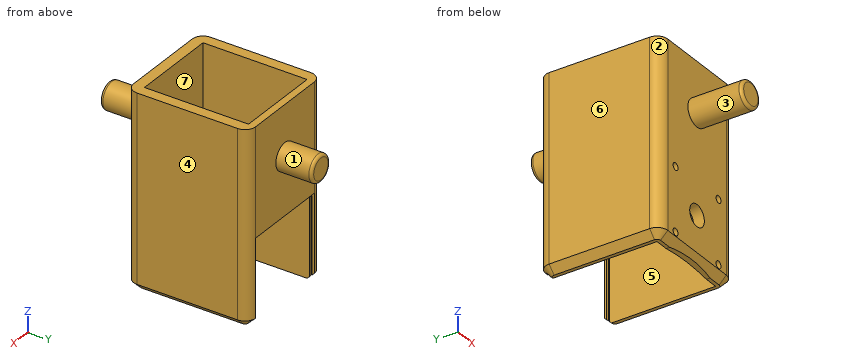
```python
from build123d import *

# Parameters (mm, degrees)
BOSS_EXTRUDE1_DEPTH = 69.85
CUT_EXTRUDE1_DEPTH  = 50.8
SKETCH3_R           = 1.27
SKETCH3_R_2         = 3.81
CUT_EXTRUDE2_DEPTH  = 50.8
SKETCH4_W           = 30.48
SKETCH4_H           = 38.1
BOSS_EXTRUDE2_DEPTH = 2.54
SKETCH5_W           = 30.48
SKETCH5_H           = 1.016
CUT_EXTRUDE3_DEPTH  = 1.016
FILLET1_R           = 3.81
SKETCH6_R           = 4.7625
BOSS_EXTRUDE3_DEPTH = 12.7
BOSS_EXTRUDE4_START = 19.05
SKETCH8_R           = 4.7625
BOSS_EXTRUDE4_DEPTH = 19.05
FILLET2_R           = 1.016
SKETCH9_W           = 38.1
SKETCH9_H           = 43.18
CUT_EXTRUDE4_DEPTH  = 2.032


# Some blends are built 0.0001 mm under size
with BuildPart() as part:
    # Sketch1 → Boss-Extrude1 (new body)
    with BuildSketch(Plane.XY):
        Polygon((15.24, -19.685), (-15.24, -19.685), (-15.24, 19.685), (-19.05, 19.685), (-19.05, -23.495), (15.24, -23.495), (19.05, -23.495), (19.05, 19.685), (15.24, 19.685), align=None)
    extrude(amount=BOSS_EXTRUDE1_DEPTH)

    # Sketch2 → Cut-Extrude1 (cut)
    with BuildSketch(Plane(origin=(0, 19.685, 0), x_dir=(1, 0, 0), z_dir=(0, 1, 0))):
        with BuildLine():
            Line((-19.05, 0), (19.05, 0))
            ThreePointArc((19.05, 0), (0, -2.54), (-19.05, 0))
        make_face()
    extrude(amount=-CUT_EXTRUDE1_DEPTH, mode=Mode.SUBTRACT)

    # Sketch3 → Cut-Extrude2 (cut)
    with BuildSketch(Plane(origin=(0, 19.685, 0), x_dir=(1, 0, 0), z_dir=(0, 1, 0))):
        with Locations(Location((-11.176, -5.842, 0), (0, 0, 270))):
            Circle(SKETCH3_R)
        with Locations(Location((11.176, -5.842, 0), (0, 0, 270))):
            Circle(SKETCH3_R)
        with Locations(Location((11.176, -28.194, 0), (0, 0, 270))):
            Circle(SKETCH3_R)
        with Locations(Location((-11.176, -28.194, 0), (0, 0, 270))):
            Circle(SKETCH3_R)
        with Locations(Location((0, -17.018, 0), (0, 0, 270))):
            Circle(SKETCH3_R_2)
    extrude(amount=-CUT_EXTRUDE2_DEPTH, mode=Mode.SUBTRACT)

    # Sketch4 → Boss-Extrude2 (add)
    with BuildSketch(Plane(origin=(0, 19.685, 0), x_dir=(1, 0, 0), z_dir=(0, 1, 0))):
        with Locations((0, -50.8)):
            Rectangle(SKETCH4_W, SKETCH4_H)
    extrude(amount=-BOSS_EXTRUDE2_DEPTH)

    # Sketch5 → Cut-Extrude3 (cut)
    with BuildSketch(Plane(origin=(-15.24, 0, 0), x_dir=(0, 0, -1), z_dir=(1, 0, 0))):
        with Locations((-15.24, 18.415)):
            Rectangle(SKETCH5_W, SKETCH5_H)
    cut_extrude3 = extrude(amount=-CUT_EXTRUDE3_DEPTH, mode=Mode.SUBTRACT)

    # Mirror1: Cut-Extrude3 across plane
    add(cut_extrude3.mirror(Plane(origin=(0, 0, 0), x_dir=(0, 0, 1), z_dir=(1, 0, 0))), mode=Mode.SUBTRACT)

    # Fillet1
    fillet1_edges = [part.edges().sort_by_distance(p)[0] for p in [
        (19.05, 19.685, 34.925),
        (19.05, -23.495, 34.925),
        (-19.05, -23.495, 34.925),
        (-19.05, 19.685, 34.925),
    ]]
    fillet(fillet1_edges, radius=FILLET1_R - 0.0001)  # a hair under: the kernel refuses the full size

    # Sketch6 → Boss-Extrude3 (add)
    with BuildSketch(Plane(origin=(0, 19.685, 0), x_dir=(1, 0, 0), z_dir=(0, 1, 0))):
        with Locations((0, -52.07)):
            Circle(SKETCH6_R)
    extrude(amount=BOSS_EXTRUDE3_DEPTH)

    # Sketch8 → Boss-Extrude4 (add)
    with BuildSketch(Plane.XZ.offset(23.495).offset(BOSS_EXTRUDE4_START)):
        with Locations((0, 52.07)):
            Circle(SKETCH8_R)
    extrude(amount=-BOSS_EXTRUDE4_DEPTH)

    # Fillet2
    fillet2_edges = [part.edges().sort_by_distance(p)[0] for p in [
        (-4.7625, 32.385, 52.07),
        (-4.7625, -42.545, 52.07),
    ]]
    fillet(fillet2_edges, radius=FILLET2_R)

    # Sketch9 → Cut-Extrude4 (cut)
    with BuildSketch(Plane(origin=(0, 0, 1.778), x_dir=(-1, 0, 0), z_dir=(0, 0, -1))):
        with Locations((0, -1.905)):
            Rectangle(SKETCH9_W, SKETCH9_H)
    extrude(amount=CUT_EXTRUDE4_DEPTH, mode=Mode.SUBTRACT)

    # Chamfer1
    # the kernel refuses this chamfer: 2.54 mm, written as the material it takes off along each edge
    with BuildSketch(Plane(origin=(-15.2401, 15.8751, 1.778), x_dir=(0, 1, 0), z_dir=(1, 0, 0))) as chamfer1_piece_1:
        with BuildLine():
            Line((1.198057951, -0.071842049), (3.881742049, 2.611842049))
            Line((3.881742049, 2.611842049), (3.932542049, 2.611842049))
            ThreePointArc((3.932542049, 2.611842049), (3.8607, 1.305921024), (3.8607, 0))
            Line((3.8607, 0), (3.8099, -0.0508))
            ThreePointArc((3.8099, -0.0508), (2.503978976, -0.0508), (1.198057951, -0.122642049))
            Line((1.198057951, -0.122642049), (1.198057951, -0.071842049))
        make_face()
    revolve(axis=Axis((-15.2401, 15.8751, 1.778), (0, 0, 1)), revolution_arc=90, mode=Mode.SUBTRACT)
    with BuildSketch(Plane(origin=(-15.2401, -19.6851, 1.778), x_dir=(-1, 0, 0), z_dir=(0, 1, 0))) as chamfer1_piece_2:
        with BuildLine():
            Line((3.881742049, 2.611842049), (1.198057951, -0.071842049))
            Line((1.198057951, -0.071842049), (1.198057951, -0.122642049))
            ThreePointArc((1.198057951, -0.122642049), (2.503978976, -0.0508), (3.8099, -0.0508))
            Line((3.8099, -0.0508), (3.8607, 0))
            ThreePointArc((3.8607, 0), (3.8607, 1.305921024), (3.932542049, 2.611842049))
            Line((3.932542049, 2.611842049), (3.881742049, 2.611842049))
        make_face()
    revolve(axis=Axis((-15.2401, -19.6851, 1.778), (0, 0, 1)), revolution_arc=90, mode=Mode.SUBTRACT)
    with BuildSketch(Plane(origin=(-19.05, 15.8751, 1.778), x_dir=(1, 0, 0), z_dir=(0, -1, 0)), Plane(origin=(19.05, -19.6851, 1.778), x_dir=(-1, 0, 0), z_dir=(0, 1, 0))) as chamfer1_piece_3:
        with BuildLine():
            Line((2.611842049, -0.071842049), (-0.071842049, 2.611842049))
            Line((-0.071842049, 2.611842049), (-0.122642049, 2.611842049))
            ThreePointArc((-0.122642049, 2.611842049), (-0.0508, 1.305921024), (-0.0508, 0))
            Line((-0.0508, 0), (0, -0.0508))
            ThreePointArc((0, -0.0508), (1.305921024, -0.0508), (2.611842049, -0.122642049))
            Line((2.611842049, -0.122642049), (2.611842049, -0.071842049))
        make_face()
    extrude(amount=35.5602, mode=Mode.SUBTRACT)
    with BuildSketch(Plane(origin=(-5.17814213, -23.495, 1.778), x_dir=(0, 0, 1), z_dir=(1, 0, 0)), Plane(origin=(-15.2401, -23.495, 1.778), x_dir=(0, 0, 1), z_dir=(1, 0, 0))) as chamfer1_piece_4:
        with BuildLine():
            Line((2.611842049, 0.071842049), (-0.071842049, -2.611842049))
            Line((-0.071842049, -2.611842049), (-0.122642049, -2.611842049))
            ThreePointArc((-0.122642049, -2.611842049), (-0.0508, -1.305921024), (-0.0508, 0))
            Line((-0.0508, 0), (0, 0.0508))
            ThreePointArc((0, 0.0508), (1.305921024, 0.0508), (2.611842049, 0.122642049))
            Line((2.611842049, 0.122642049), (2.611842049, 0.071842049))
        make_face()
    extrude(amount=20.41824213, mode=Mode.SUBTRACT)
    with BuildSketch(Plane(origin=(15.2401, 15.8751, 1.778), x_dir=(1, 0, 0), z_dir=(0, -1, 0))) as chamfer1_piece_5:
        with BuildLine():
            Line((1.198057951, -0.071842049), (3.881742049, 2.611842049))
            Line((3.881742049, 2.611842049), (3.932542049, 2.611842049))
            ThreePointArc((3.932542049, 2.611842049), (3.8607, 1.305921024), (3.8607, 0))
            Line((3.8607, 0), (3.8099, -0.0508))
            ThreePointArc((3.8099, -0.0508), (2.503978976, -0.0508), (1.198057951, -0.122642049))
            Line((1.198057951, -0.122642049), (1.198057951, -0.071842049))
        make_face()
    revolve(axis=Axis((15.2401, 15.8751, 1.778), (0, 0, 1)), revolution_arc=90, mode=Mode.SUBTRACT)
    with BuildSketch(Plane(origin=(15.2401, -19.6851, 1.778), x_dir=(0, -1, 0), z_dir=(-1, 0, 0))) as chamfer1_piece_6:
        with BuildLine():
            Line((1.198057951, -0.071842049), (3.881742049, 2.611842049))
            Line((3.881742049, 2.611842049), (3.932542049, 2.611842049))
            ThreePointArc((3.932542049, 2.611842049), (3.8607, 1.305921024), (3.8607, 0))
            Line((3.8607, 0), (3.8099, -0.0508))
            ThreePointArc((3.8099, -0.0508), (2.503978976, -0.0508), (1.198057951, -0.122642049))
            Line((1.198057951, -0.122642049), (1.198057951, -0.071842049))
        make_face()
    revolve(axis=Axis((15.2401, -19.6851, 1.778), (0, 0, 1)), revolution_arc=90, mode=Mode.SUBTRACT)
    with BuildSketch(Plane(origin=(15.2401, 19.685, 1.778), x_dir=(0, -1, 0), z_dir=(-1, 0, 0)), Plane(origin=(0.436979495, 19.685, 1.778), x_dir=(0, -1, 0), z_dir=(-1, 0, 0))) as chamfer1_piece_7:
        with BuildLine():
            Line((2.611842049, -0.071842049), (-0.071842049, 2.611842049))
            Line((-0.071842049, 2.611842049), (-0.122642049, 2.611842049))
            ThreePointArc((-0.122642049, 2.611842049), (-0.0508, 1.305921024), (-0.0508, 0))
            Line((-0.0508, 0), (0, -0.0508))
            ThreePointArc((0, -0.0508), (1.305921024, -0.0508), (2.611842049, -0.122642049))
            Line((2.611842049, -0.122642049), (2.611842049, -0.071842049))
        make_face()
    extrude(amount=15.677079495, mode=Mode.SUBTRACT)


solid = part.part
```
Part model, mm, in its own coordinate system. Face numbers are marked on the shaded views. A direction names the side the tool comes from. Round coordinates to 2 decimals unless told otherwise and drop trailing zeros. Write each loop counter-clockwise with the first axis right and the second up, starting at its lowest first coordinate (ties: lowest second). Pieces come first, ordered by that corner, then holes. Notation, with made-up numbers: (-14, -35.5) -> (12, -35.5) arc R32 cw to (12, 1.5) -> close; hole circle Ø9 at (75, 19.5). An arc over 180 degrees is marked (long way). Return JSON: item names as keys, results as strings. Group by question number.
Q1. Which spindle directions (+Z, -Z, +X, -X, +Y, -Y) get a long thin tool onto all of the face, cutting with end or side? Do the marked faces 1, 2 and 3. Say none if no direction does.
Q2. Saw through at C-C on y = 8.5. Write the cut outline in (x, z).
Q3. Probe L1, parallel to X at y = 10, z = 35.5; L2, parallel to Y at x = -13, z = 60 (3 decimals); L3, parallel to Y at x = -12, z = 15 (3 decimals). List the from-to ranges inside material, lowest first. Write a range as [from, to].
Q4. Mould opens along X. For the marked faces 4, 5, 6 and 7 say: pulls with the +X half, pulls with the -X half, needs draft (parallel to the pull), parting line crosses it, or undercut.
Q5. Saw through at A-A on z = 45. Write the cut outline in (x, y) (3 decimals), plus the area to 3 significant figures.
Q6. Saw through at B-B on x = 0. State how many separate pieces and enclosed holes the cut face has, plus the area to 3 significant figures.
Q7. Pin check, flat tips, straight feed: pin 1 (0.8 mm diameter, centred on x = -15.5, z = 23.5, fed in from -Y) (3 decimals); pin 2 (0.8 mm diameter, centred on x = 16, z = 13, fed in from +Y); pin 3 (1.5 mm diameter, centred on x = 11.176, z = 5.842, fed in from +Y); pin 4 (0.8 mm diameter, centred on y = 18.5, z = 17, fed in from -X). Stop position of each tip, or through.
Answer:
{
 "1": {"face 1": "+Y", "face 2": "+Z, -Z, -X, -Y", "face 3": "-Y"},
 "2": {"outline": "(-19.05, 4.32) -> (-16.51, 1.78) -> (-15.24, 1.78) -> (-15.24, 69.85) -> (-19.05, 69.85) -> close; (15.24, 1.78) -> (16.51, 1.78) -> (19.05, 4.32) -> (19.05, 69.85) -> (15.24, 69.85) -> close"},
 "3": {"L1": "[-19.05, -15.24], [15.24, 19.05]", "L2": "[-23.495, -19.685], [17.145, 19.685]", "L3": "[-23.495, -19.685]"},
 "4": {"face 4": "pulls with the +X half", "face 5": "undercut", "face 6": "pulls with the -X half", "face 7": "undercut"},
 "5": {"outline": "(-19.05, -19.685) arc R3.81 ccw to (-15.24, -23.495) -> (15.24, -23.495) arc R3.81 ccw to (19.05, -19.685) -> (19.05, 15.875) arc R3.81 ccw to (15.24, 19.685) -> (-15.24, 19.685) arc R3.81 ccw to (-19.05, 15.875) -> close; hole (-15.24, -19.685) -> (15.24, -19.685) -> (15.24, 17.145) -> (-15.24, 17.145) -> close", "area": "510 mm2"},
 "6": {"separate pieces": "3", "enclosed holes": "0", "area": "624 mm2"},
 "7": {"pin 1": "y = -23.495", "pin 2": "y = 19.67", "pin 3": "through", "pin 4": "x = -18.33"}
}
